from build123d import *
from build123d.topology import SkipClean

# Parameters (mm, degrees)
SKETCH1_R           = 27.5
BOSS_EXTRUDE1_DEPTH = 24
CUT_EXTRUDE3_START  = -2
CUT_EXTRUDE3_DEPTH  = 48.700109409
CIRPATTERN1_COUNT   = 6
CUT_EXTRUDE4_DEPTH  = 24
CIRPATTERN2_COUNT   = 6
CUT_EXTRUDE5_DEPTH  = 8.8
SKETCH6_R           = 1.9
CUT_EXTRUDE6_DEPTH  = 24


with BuildPart() as part:
    # Sketch1 → Boss-Extrude1 (new body)
    with BuildSketch(Plane(origin=(0, 0, 0), x_dir=(1, 0, 0), z_dir=(0, 1, 0))):
        with Locations(Location((0, 0, 0), (0, 0, 270))):
            Circle(SKETCH1_R)
    extrude(amount=BOSS_EXTRUDE1_DEPTH)

    # Sketch2 → Cut-Extrude3 (cut)
    with BuildSketch(Plane(origin=(0, 0, 0), x_dir=(1, 0, 0), z_dir=(0, 1, 0)).offset(CUT_EXTRUDE3_START)):
        with BuildLine():
            Line((-3, 27.335873866), (-4, 24.171263931))
            ThreePointArc((-4, 24.171263931), (0, 24.5), (4, 24.171263931))
            Line((4, 24.171263931), (3, 27.335873866))
            ThreePointArc((3, 27.335873866), (0, 27.5), (-3, 27.335873866))
        make_face()
    cut_extrude3 = extrude(amount=CUT_EXTRUDE3_DEPTH, mode=Mode.SUBTRACT)

    # CirPattern1: Cut-Extrude3 ×6 about axis
    cirpattern1_axis = Axis((0, 0, 0), (0, 1, 0))
    for i in range(1, CIRPATTERN1_COUNT):
        add(cut_extrude3.rotate(cirpattern1_axis, i * 360 / CIRPATTERN1_COUNT), mode=Mode.SUBTRACT)

    # Sketch3 → Cut-Extrude4 (cut)
    with BuildSketch(Plane(origin=(0, 0, 0), x_dir=(1, 0, 0), z_dir=(0, 1, 0))):
        with BuildLine():
            ThreePointArc((19.52562419, 9), (13.682742888, 16.584105253), (5.126758988, 20.879807046))
            Line((5.126758988, 20.879807046), (-1.732050808, 9))
            Line((-1.732050808, 9), (19.52562419, 9))
        make_face()
    cut_extrude4 = extrude(amount=CUT_EXTRUDE4_DEPTH, mode=Mode.SUBTRACT)

    # CirPattern2: Cut-Extrude4 ×6 about axis
    cirpattern2_axis = Axis((0, 0, 0), (0, 1, 0))
    for i in range(1, CIRPATTERN2_COUNT):
        add(cut_extrude4.rotate(cirpattern2_axis, i * 360 / CIRPATTERN2_COUNT), mode=Mode.SUBTRACT)

    # Sketch5 → Cut-Extrude5 (cut)
    with BuildSketch(Plane(origin=(0, 24, 0), x_dir=(1, 0, 0), z_dir=(0, 1, 0))):
        Polygon((0, 6.92820323), (-6, 3.464101615), (-6, -3.464101615), (0, -6.92820323), (6, -3.464101615), (6, 3.464101615), align=None)
    cut_extrude5 = extrude(amount=-CUT_EXTRUDE5_DEPTH, mode=Mode.SUBTRACT)

    # Sketch6 → Cut-Extrude6 (cut)
    with BuildSketch(Plane(origin=(0, 0, 0), x_dir=(1, 0, 0), z_dir=(0, 1, 0))):
        with Locations(Location((0, 0, 0), (0, 0, 270))):
            Circle(SKETCH6_R)
    extrude(amount=CUT_EXTRUDE6_DEPTH, mode=Mode.SUBTRACT)

    # Mirror1: Cut-Extrude5 across plane
    add(cut_extrude5.mirror(Plane.ZX.offset(12)), mode=Mode.SUBTRACT)

    # Sketch7 → Cut-Revolve1 (revolve, cut)
    with SkipClean():  # the faces are left unmerged after this step: merging them gives an invalid solid
        with BuildSketch(Plane.XY, mode=Mode.PRIVATE) as cut_revolve1_sk:
            Polygon((24.5, 12), (24.5, 14), (27.5, 16), (27.5, 12), align=None)
        cut_revolve1 = revolve(cut_revolve1_sk.sketch.rotate(Axis((0, 24, 0), (0, -1, 0)), 270), axis=Axis((0, 24, 0), (0, -1, 0)), mode=Mode.SUBTRACT)

    # Mirror2: Cut-Revolve1 across plane
    with SkipClean():  # the faces are left unmerged after this step: merging them gives an invalid solid
        add(cut_revolve1.mirror(Plane.ZX.offset(12)), mode=Mode.SUBTRACT)


solid = part.part
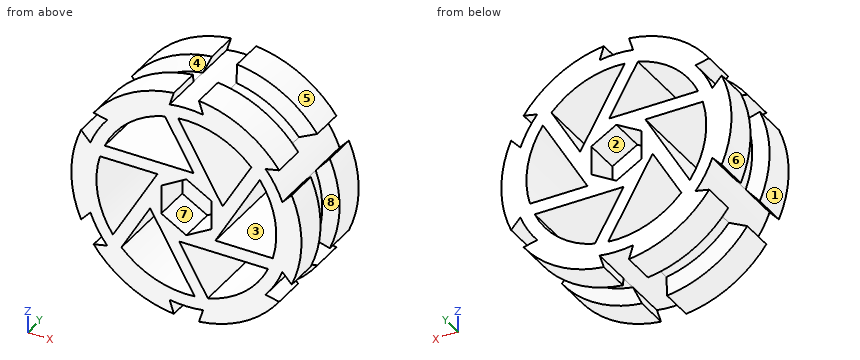
Can you work these out from the model? Positions are in its coordinate system, mm. Face numbers are marked on the shaded views. A direction names the side the tool comes from. Give positions to 0.01 mm unless a question says otherwise; leave off trailing zeros. Order: outer loops, then holes, each group sorted by start corner. A loop starts at its lowest first (then second) coordinate and runs counter-clockwise, first axis right, second up. Notation, with made-up numbers: M 19,-27.75 L 42,-27.75 A7 cw 42,-17.75 Z; hole C 61.25,-14.75 d8. An arc over 180 degrees is marked long. Use one line per item in the form item = value. Start each with the question number.
Item 1: For the marked faces 1, 2, 3, 4 and 5, which set-ups out of +Z, -Z, +X, -X, +Y, -Y let a thin tool reach every point of the face, with its end or its side?
Item 2: If we section it at B-B (z = 0): State how many separate pieces and enclosed holes the cut face has, then the cut area to 3 significant figures.
Item 3: If we section it at A-A (y = 13): Write out the boundary of the cut face in (x, z), then the cut area to 3 significant figures.
Item 4: We'd pull the mould along X, two halves only. Please class the marked faces 6, 7 and 8: +X half, -X half, draft (parallel to the pull), parting line (faces both ways), or undercut.
Item 5: If I drill on line 1 along X through (y, z) = (9.5, 18.5); line 2 along X through (y, z) = (5, -17); line 3 along Z through (x, y) = (14.5, 15), over which ranges is the centre line in solid material (lowest first)?
Item 6: Will these pins go through, and if not, where does the flat tip stop? pin 1 Ø7 at (x, y) = (12.5, 9) entering from +Z; pin 2 Ø6 at (x, z) = (-2, 2) entering from -Y; pin 3 Ø1.5 at (y, z) = (4, 7.5) entering from -X.
Outcome:
q1.face_1 = -X, +Y, -Y
q1.face_2 = +Y
q1.face_3 = +Y, -Y
q1.face_4 = +Z, -X
q1.face_5 = +Z, +X, +Y, -Y
q2.separate_pieces = 4
q2.enclosed_holes = 0
q2.area = 515 mm2
q3.outline = C 0,0 d49; hole M -20.65,6 A21.5 ccw -17.56,-12.41 L -6.93,6 Z; hole M -19.53,9 L 1.73,9 L -5.13,20.88 A21.5 ccw Z; hole M -15.52,-14.88 A21.5 ccw 1.97,-21.41 L -8.66,-3 Z; hole M -1.97,21.41 L 8.66,3 L 15.52,14.88 A21.5 ccw Z; hole C 0,0 d3.8; hole M -1.73,-9 L 5.13,-20.88 A21.5 ccw 19.53,-9 Z; hole M 6.93,-6 L 20.65,-6 A21.5 ccw 17.56,12.41 Z
q3.area = 956 mm2
q4.face_6 = -X half
q4.face_7 = undercut
q4.face_8 = +X half
q5.line_1 = -17.18 to -10.95, -3.75 to -0.29, 10.95 to 17.18
q5.line_2 = -21.62 to -13.16, -0.58 to 2.89, 13.16 to 21.62
q5.line_3 = -21.58 to -15.87, -9 to -6, 7.11 to 13.11, 15.87 to 21.58
q6.pin_1 = 25.93
q6.pin_2 = 8.8
q6.pin_3 = -26.66
